```python
from build123d import *

# Parameters (mm, degrees)
BOSS_EXTRUDE1_DEPTH = 3.999992
CUT_EXTRUDE1_DEPTH  = 1.999996
CUT_EXTRUDE2_REACH  = 56
CUT_EXTRUDE3_DEPTH  = 3.703193
CUT_EXTRUDE4_DEPTH  = 2.999994
SKETCH6_R           = 0.621776252
CUT_EXTRUDE5_DEPTH  = 41.509250857
CUT_EXTRUDE6_DEPTH  = 2.999994


with BuildPart() as part:
    # Sketch1 → Boss-Extrude1 (new body)
    with BuildSketch(Plane(origin=(0, 0, 0), x_dir=(1, 0, 0), z_dir=(0, 1, 0))):
        with BuildLine():
            Line((-14.9999954, -19.9999981), (14.9999954, -19.9999981))
            ThreePointArc((14.9999954, -19.9999981), (34.9999935, 0), (14.9999954, 19.9999981))
            Line((14.9999954, 19.9999981), (-14.9999954, 19.9999981))
            Line((-14.9999954, 19.9999981), (-14.9999954, -19.9999981))
        make_face()
    extrude(amount=BOSS_EXTRUDE1_DEPTH)

    # Sketch2 → Cut-Extrude1 (cut)
    with BuildSketch(Plane(origin=(0, 3.999992, 0), x_dir=(1, 0, 0), z_dir=(0, 1, 0))):
        Polygon((-14.9999954, -16.7499919), (-14.9999954, -13.2499989), (-12.9999994, -13.2499989), (-12.9999994, -12.0500013), (-10.0000054, -12.0500013), (-10.0000054, -13.2499989), (-2.999994, -13.2499989), (-2.999994, -16.7499919), (-10.0000054, -16.7499919), (-10.0000054, -17.9499895), (-12.9999994, -17.9499895), (-12.9999994, -16.7499919), align=None)
        Polygon((-14.9999954, 16.7499919), (-12.9999994, 16.7499919), (-12.9999994, 17.9499895), (-10.0000054, 17.9499895), (-10.0000054, 16.7499919), (-2.999994, 16.7499919), (-2.999994, 13.2499989), (-10.0000054, 13.2499989), (-10.0000054, 12.0500013), (-12.9999994, 12.0500013), (-12.9999994, 13.2499989), (-14.9999954, 13.2499989), align=None)
    extrude(amount=-CUT_EXTRUDE1_DEPTH, mode=Mode.SUBTRACT)

    # Cut-Extrude2: up to this face of the body (flat: up to its plane)
    cut_extrude2_end = Plane(part.part.faces().sort_by_distance((-2.999994, 2.999994, -14.9999954))[0])
    # Sketch3 → Cut-Extrude2 (cut, up to the picked face)
    with BuildSketch(Plane.ZY.offset(14.9999954), mode=Mode.PRIVATE) as cut_extrude2_sk1:
        with BuildLine():
            Line((13.2499989, 1.999996), (16.7499919, 1.999996))
            ThreePointArc((16.7499919, 1.999996), (14.9999954, 0.2499995), (13.2499989, 1.999996))
        make_face()
    cut_extrude2_tool1 = split(extrude(cut_extrude2_sk1.sketch, amount=-CUT_EXTRUDE2_REACH, mode=Mode.PRIVATE), bisect_by=cut_extrude2_end, keep=Keep.BOTH, mode=Mode.PRIVATE)
    # Sketch3 → Cut-Extrude2 (cut, up to the picked face)
    with BuildSketch(Plane.ZY.offset(14.9999954), mode=Mode.PRIVATE) as cut_extrude2_sk2:
        with BuildLine():
            Line((-13.2499989, 1.999996), (-16.7499919, 1.999996))
            ThreePointArc((-16.7499919, 1.999996), (-14.9999954, 0.2499995), (-13.2499989, 1.999996))
        make_face()
    cut_extrude2_tool2 = split(extrude(cut_extrude2_sk2.sketch, amount=-CUT_EXTRUDE2_REACH, mode=Mode.PRIVATE), bisect_by=cut_extrude2_end, keep=Keep.BOTH, mode=Mode.PRIVATE)
    add(cut_extrude2_tool1.solids().sort_by(Axis((-14.999995, 1.257274, 14.999995), (1, 0, 0)))[0], mode=Mode.SUBTRACT)
    add(cut_extrude2_tool2.solids().sort_by(Axis((-14.999995, 1.257274, -14.999995), (1, 0, 0)))[0], mode=Mode.SUBTRACT)

    # Sketch4 → Cut-Extrude3 (cut)
    with BuildSketch(Plane(origin=(0, 3.999992, 0), x_dir=(1, 0, 0), z_dir=(0, 1, 0))):
        Polygon((-12.9999994, 13.2499989), (-12.9999994, 12.0500013), (-10.0000054, 12.0500013), (-10.0000054, 13.2499989), (-10.0000054, 16.7499919), (-10.0000054, 17.9499895), (-12.9999994, 17.9499895), (-12.9999994, 16.7499919), align=None)
        Polygon((-10.0000054, -16.7499919), (-10.0000054, -13.2499989), (-10.0000054, -12.0500013), (-12.9999994, -12.0500013), (-12.9999994, -13.2499989), (-12.9999994, -16.7499919), (-12.9999994, -17.9499895), (-10.0000054, -17.9499895), align=None)
    extrude(amount=-CUT_EXTRUDE3_DEPTH, mode=Mode.SUBTRACT)

    # Sketch5 → Cut-Extrude4 (cut)
    with BuildSketch(Plane.ZY.offset(10.0000054)):
        Polygon((-17.4419895, 0), (-12.5580013, 0), (-12.0500013, 0.3048), (-17.9499895, 0.3048), align=None)
        Polygon((12.5580013, 0), (12.0500013, 0.3048), (17.9499895, 0.3048), (17.4419895, 0), align=None)
    extrude(amount=CUT_EXTRUDE4_DEPTH, mode=Mode.SUBTRACT)

    # Sketch6 → Cut-Extrude5 (cut, through all)
    with BuildSketch(Plane(origin=(0, 3.999992, 0), x_dir=(1, 0, 0), z_dir=(0, 1, 0))):
        with BuildLine():
            ThreePointArc((18.60506983, 0.504260657), (19.593270199, 0.000879919), (18.60506983, -0.502500819))
            ThreePointArc((18.60506983, -0.502500819), (14.9999954, -3.639168681), (11.39492097, -0.502500819))
            ThreePointArc((11.39492097, -0.502500819), (10.406720601, 0.000879919), (11.39492097, 0.504260657))
            ThreePointArc((11.39492097, 0.504260657), (14.9999954, 3.640928519), (18.60506983, 0.504260657))
        make_face()
        with Locations(Location((9.040415251, 0.000347085, 0), (0, 0, 270))):
            Circle(SKETCH6_R)
        with Locations(Location((7.051800737, 0.000347085, 0), (0, 0, 270))):
            Circle(SKETCH6_R)
        with Locations(Location((5.063186223, 0.000347085, 0), (0, 0, 270))):
            Circle(SKETCH6_R)
        with Locations(Location((3.074571709, 0.000347085, 0), (0, 0, 270))):
            Circle(SKETCH6_R)
        with Locations(Location((1.085957195, 0.000347085, 0), (0, 0, 270))):
            Circle(SKETCH6_R)
        with Locations(Location((20.959575549, 0.000347085, 0), (0, 0, 270))):
            Circle(SKETCH6_R)
        with Locations(Location((22.948190063, 0.000347085, 0), (0, 0, 270))):
            Circle(SKETCH6_R)
        with Locations(Location((24.936804577, 0.000347085, 0), (0, 0, 270))):
            Circle(SKETCH6_R)
        with Locations(Location((26.925419091, 0.000347085, 0), (0, 0, 270))):
            Circle(SKETCH6_R)
        with Locations(Location((28.914033605, 0.000347085, 0), (0, 0, 270))):
            Circle(SKETCH6_R)
    extrude(amount=-CUT_EXTRUDE5_DEPTH, mode=Mode.SUBTRACT)

    # Sketch7 → Cut-Extrude6 (cut)
    with BuildSketch(Plane(origin=(0, 3.999992, 0), x_dir=(1, 0, 0), z_dir=(0, 1, 0))):
        with BuildLine():
            Line((0.7589266, 2.237934119), (14.5982182, 3.734679919))
            ThreePointArc((14.5982182, 3.734679919), (14.9999954, 3.75634324), (15.4017726, 3.734679919))
            Line((15.4017726, 3.734679919), (29.2410642, 2.237934119))
            ThreePointArc((29.2410642, 2.237934119), (31.249997536, 0.000879919), (29.2410642, -2.236174281))
            Line((29.2410642, -2.236174281), (15.4017726, -3.732920081))
            ThreePointArc((15.4017726, -3.732920081), (14.9999954, -3.754583403), (14.5982182, -3.732920081))
            Line((14.5982182, -3.732920081), (0.7589266, -2.236174281))
            ThreePointArc((0.7589266, -2.236174281), (-1.250006736, 0.000879919), (0.7589266, 2.237934119))
        make_face()
    extrude(amount=-CUT_EXTRUDE6_DEPTH, mode=Mode.SUBTRACT)


solid = part.part
```
CAD build for the part. Positions are in the model's coordinates, mm. A direction names the side the tool comes from. Round coordinates to 2 decimals unless told otherwise and drop trailing zeros. Loops run counter-clockwise (first coordinate to the right, second up) from the corner with the lowest first, then second, coordinate; pieces in that order, holes last. Notation, with made-up numbers: (44, 86) - (79, 86) arc R24 cw to (79, 96) - close; hole circle Ø10 at (-3.5, 74). An arc over 180 degrees is marked (long way). Return JSON: item names as keys, results as strings. Group by question number.
Q1. Flat gauge pins, fed straight in: pin 1 Ø1.1 at (x, z) = (9.04, 0) entering from +Y; pin 2 Ø1.6 at (x, z) = (11.03, 0) entering from +Y. Where does each tip first touch, or does it go through?
Q2. Drill centre lines: line 1 along Z through (x, y) = (-11.5, 1.65); line 2 along Z through (x, y) = (-7, 3.6); line 3 along Z through (x, y) = (17, 0.4). Where is each one in solid material? Low to high. Write a range as [from, to].
Q3. Band-saw the part on B-B on z = -9. Give the cut face in (x, y).
Q4. Two-plate mould, pull along X, no slides. Class faces 4 (the face through (-3, 2, -15)), 5 (the face through (-13, 0.7, 16.4)), 6 (the face through (-14, 3, -13.25)): +X half, -X half, draft (parallel to the pull), parting line (faces both ways), or undercut.
Q5. Tool access for faces 1 (the face through (14.93, 0.51, -3.64)), 2 (the face through (19, 1, 1)), 3 (the face through (-14.01, 0.25, 15.04)): list every direction of +Z, -Z, +X, -X, +Y, -Y with a clear straight run to the whole face (end or side of a thin tool).
Q6. Band-saw the part on A-A on z = 6.5. Give the cut face in (x, y), plus the area to 3 significant figures.
Solutions:
{
 "1": {"pin 1": "passes through", "pin 2": "stops at y = 1"},
 "2": {"line 1": "z = [-20, -17.95], [-12.05, 12.05], [17.95, 20]", "line 2": "z = [-20, -16.75], [-13.25, 13.25], [16.75, 20]", "line 3": "z = [-19.9, -3.04], [3.04, 19.9]"},
 "3": {"outline": "(-15, 0) - (32.86, 0) - (32.86, 4) - (-15, 4) - close"},
 "4": {"face 4": "-X half", "face 5": "undercut", "face 6": "draft"},
 "5": {"face 1": "+Y, -Y", "face 2": "+Y", "face 3": "-X, +Y"},
 "6": {"outline": "(-15, 0) - (33.91, 0) - (33.91, 4) - (-15, 4) - close", "area": "196 mm^2"}
}
